from build123d import *

# Parameters (mm, degrees)
SKETCH1_R                                       = 15
SKETCH1_R_2                                     = 10
BOSS_EXTRUDE1_DEPTH                             = 1.5
CSK_FOR_M2_FLAT_HEAD_MACHINE_SCREW1_D           = 2.4
CSK_FOR_M2_FLAT_HEAD_MACHINE_SCREW1_CSINK_D     = 4.4
CSK_FOR_M2_FLAT_HEAD_MACHINE_SCREW1_CSINK_ANGLE = 90
CIRPATTERN1_COUNT                               = 6


with BuildPart() as part:
    # Sketch1 → Boss-Extrude1 (new, symmetric)
    with BuildSketch(Plane(origin=(0, 0, 0), x_dir=(1, 0, 0), z_dir=(0, 1, 0))):
        with Locations(Location((0, 0, 0), (0, 0, 270))):
            Circle(SKETCH1_R)
        with Locations(Location((0, 0, 0), (0, 0, 270))):
            Circle(SKETCH1_R_2, mode=Mode.SUBTRACT)
    extrude(amount=BOSS_EXTRUDE1_DEPTH, both=True)

    # CSK for M2 Flat Head Machine Screw1 (through all)
    with Locations(Plane(origin=(0, 1.5, -12.5), x_dir=(0, 0, 1), z_dir=(0, 1, 0))):
        with Locations((0, 0)):
            csk_for_m2_flat_head_machine_screw1 = CounterSinkHole(CSK_FOR_M2_FLAT_HEAD_MACHINE_SCREW1_D / 2, CSK_FOR_M2_FLAT_HEAD_MACHINE_SCREW1_CSINK_D / 2, counter_sink_angle=CSK_FOR_M2_FLAT_HEAD_MACHINE_SCREW1_CSINK_ANGLE)

    # CirPattern1: CSK for M2 Flat Head Machine Screw1 ×6 about axis
    cirpattern1_axis = Axis((0, 0, 0), (0, 1, 0))
    for i in range(1, CIRPATTERN1_COUNT):
        add(csk_for_m2_flat_head_machine_screw1.rotate(cirpattern1_axis, i * 360 / CIRPATTERN1_COUNT), mode=Mode.SUBTRACT)


solid = part.part
Part model, mm, in its own coordinate system. Give positions to 0.01 mm unless a question says otherwise; leave off trailing zeros. Loops run counter-clockwise (first coordinate to the right, second up) from the corner with the lowest first, then second, coordinate; pieces in that order, holes last.
(1) Drill centre lines: line 1 along X through (y, z) = (-0.45, 6.25); line 2 along X through (y, z) = (1.4, 6.75); line 3 along X through (y, z) = (0.5, 0). Where is each one in solid material? Low to high.
Return value:
line 1: x = -13.64 to -12.03, -9.63 to -7.81, 7.81 to 9.63, 12.03 to 13.64
line 2: x = -13.4 to -12.86, -8.79 to -7.38, 7.38 to 8.79, 12.86 to 13.4
line 3: x = -15 to -10, 10 to 15
(2) Band-saw the part on B-B (z = 1.25). Write the cut outline in (x, y), and give its area (3 significant figures).
Return value:
outline: (-14.95, -1.5) - (-9.92, -1.5) - (-9.92, 1.5) - (-14.95, 1.5) - close; (9.92, -1.5) - (14.95, -1.5) - (14.95, 1.5) - (9.92, 1.5) - close
area: 30.2 mm2
(3) Pin check, flat tips, straight feed: pin 1 (4 mm diameter, centred on x = -10.83, z = -6.25, fed in from +Y); pin 2 (3 mm diameter, centred on x = 10.83, z = -6.25, fed in from -Y); pin 3 (1.5 mm diameter, centred on x = -4, y = -0.5, fed in from -Z); pin 4 (1.5 mm diameter, centred on x = 1, y = -0.5, fed in from -Z). Stop position of each tip, or through.
Return value:
pin 1: stops at y = 1.3
pin 2: stops at y = -1.5
pin 3: stops at z = -14.64
pin 4: stops at z = -15
(4) Band-saw the part on A-A (x = 0). Write the cut outline in (y, z), and give its area (3 significant figures).
Return value:
outline: (-1.5, -15) - (1.5, -15) - (1.5, -14.7) - (0.5, -13.7) - (-1.5, -13.7) - close; (-1.5, -11.3) - (0.5, -11.3) - (1.5, -10.3) - (1.5, -10) - (-1.5, -10) - close; (-1.5, 10) - (1.5, 10) - (1.5, 10.3) - (0.5, 11.3) - (-1.5, 11.3) - close; (-1.5, 13.7) - (0.5, 13.7) - (1.5, 14.7) - (1.5, 15) - (-1.5, 15) - close
area: 13.6 mm2
(5) Pull direction Z, two halves, no side cores. Call faces 1 (the flat face through (-3, 1.5, 10)), 2 (the cylindrical face through (12, -0.5, -6.5)), 3 (the cylindrical face through (0.66, 0.021, -14.985)): pulls with the +Z half, pulls with the -Z half, needs draft (parallel to the pull), parting line crosses it, or undercut.
Return value:
face 1: needs draft
face 2: undercut
face 3: parting line crosses it
(6) Band-saw the part on D-D (y = -0.1). Write the cut outline in (x, z).
Return value:
outline: circle Ø30 at (0, 0); hole circle Ø2.4 at (-10.83, -6.25); hole circle Ø2.4 at (-10.83, 6.25); hole circle Ø20 at (0, 0); hole circle Ø2.4 at (0, -12.5); hole circle Ø2.4 at (0, 12.5); hole circle Ø2.4 at (10.83, -6.25); hole circle Ø2.4 at (10.83, 6.25)
(7) Band-saw the part on C-C (x = 8.25). Write the cut outline in (y, z), and give its area (3 significant figures).
Return value:
outline: (-1.5, -12.53) - (1.5, -12.53) - (1.5, -5.65) - (-1.5, -5.65) - close; (-1.5, 5.65) - (1.5, 5.65) - (1.5, 12.53) - (-1.5, 12.53) - close
area: 41.3 mm2
